Here's how the part is built. I have some questions about the finished solid (model axes, mm). Face numbers are marked on the shaded views. Coordinates: 2 decimals unless noted, no trailing zeros. Write each loop counter-clockwise with the first axis right and the second up, starting at its lowest first coordinate (ties: lowest second). Pieces come first, ordered by that corner, then holes.
Item 1: We'd pull the mould along X, two halves only. Please class the marked faces 1, 2, 3 and 4: +X half, -X half, draft (parallel to the pull), parting line (faces both ways), or undercut.
Item 2: If we section it at D-D (y = 10): Please give me the cut outline in (x, z), then the cut area to 3 significant figures.
Item 3: If I drill on line 1 (X direction, y = 44, z = 36); line 2 (Y direction, x = -1.5, z = 21); line 3 (Z direction, x = -0.25, y = 27.5), over which ranges is the centre line in solid material (lowest first)?
Item 4: If we section it at A-A (x = -2): Please give me the cut outline in (y, z), then the cut area to 3 significant figures.
Item 5: I'm going to push flat-ended pins straight in: pin 1 Ø6 at (x, z) = (-3, 32) entering from -Y; pin 2 Ø4 at (x, y) = (-2, 12) entering from +Z; pin 3 Ø2 at (x, z) = (3, 19.5) entering from -Y. Where does each tip first touch, or does it pass through?
Item 6: If we section it at C-C (z = 43): Please give me the cut outline in (x, y), then the cut area to 3 significant figures.
Item 7: If we section it at B-B (y = 16.5): Please give me the cut outline in (x, z).
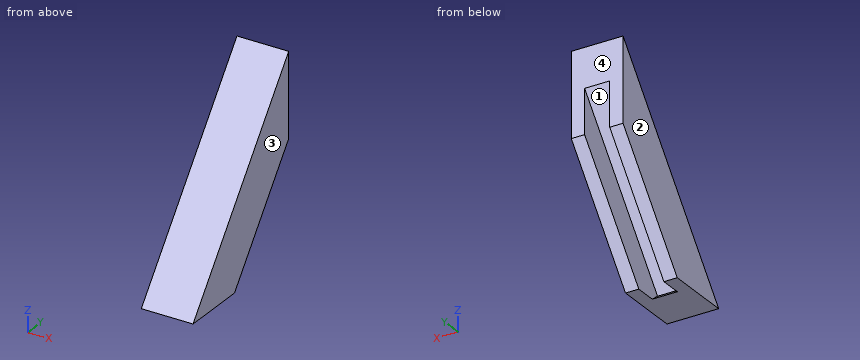
from build123d import *

# Parameters (mm, degrees)
F1_DEPTH      = 7.9375
F4_W          = 7.6985172927
F4_H          = 8.837191388
F5_DEPTH      = 32.041668515
F5_DEPTH_BACK = 25.4


with BuildPart() as f1:
    # F6 (on Right) → F1 (new body, symmetric)
    with BuildSketch(Plane.YZ):
        Polygon((46.5895857938, 59.2058200122), (0, 0), (20.2007462682, 0), (46.5895857938, 33.5348094786), align=None)
    extrude(amount=F1_DEPTH, both=True)

    # F4 (on face) → F5 (cut, two sides)
    with BuildSketch(Plane(origin=(0, 20.9196058881, 26.5845338574), x_dir=(1, 0, 0), z_dir=(0, -0.6184018342, -0.7858620562))) as f5_sk:
        with Locations((0, -11.8702491745)):
            Rectangle(F4_W, F4_H)
    extrude(amount=-F5_DEPTH, mode=Mode.SUBTRACT)
    extrude(f5_sk.sketch, amount=F5_DEPTH_BACK, mode=Mode.SUBTRACT)


solid = f1.part
Answer list:
1. face 1: undercut
1. face 2: -X half
1. face 3: +X half
1. face 4: draft
2. outline: (-7.94, 0) - (7.94, 0) - (7.94, 12.71) - (-7.94, 12.71) - close
2. area: 202 mm2
3. line 1: x = -7.94 to -3.85, 3.85 to 7.94
3. line 2: y = 16.53 to 26.01
3. line 3: z = 22.9 to 34.95
4. outline: (0, 0) - (13.63, 0) - (11.07, 2.02) - (46.59, 47.16) - (46.59, 59.21) - close
4. area: 508 mm2
5. pin 1: stops at y = 22.82
5. pin 2: stops at z = 17.79
5. pin 3: stops at y = 14.56
6. outline: (-7.94, 33.84) - (7.94, 33.84) - (7.94, 46.59) - (3.85, 46.59) - (3.85, 43.32) - (-3.85, 43.32) - (-3.85, 46.59) - (-7.94, 46.59) - close
6. area: 177 mm2
7. outline: (-7.94, 0) - (-3.85, 0) - (-3.85, 8.92) - (3.85, 8.92) - (3.85, 0) - (7.94, 0) - (7.94, 20.97) - (-7.94, 20.97) - close
